Check sheet for the drawn part. Datum: minimum x, y, z corner. Units: mm. A direction names the side the tool comes from. Give positions to 0.01 mm unless a question says otherwise; leave off trailing zeros. Write each loop counter-clockwise with the first axis right and the second up, starting at its lowest first coordinate (ties: lowest second). Pieces come first, ordered by that corner, then holes. Notation, with made-up numbers: M 84,55.5 L 108,55.5 A28 ccw 108,90.5 Z; hole C -13,-27 d4. An arc over 180 degrees is marked long. Write item = value, one per line.
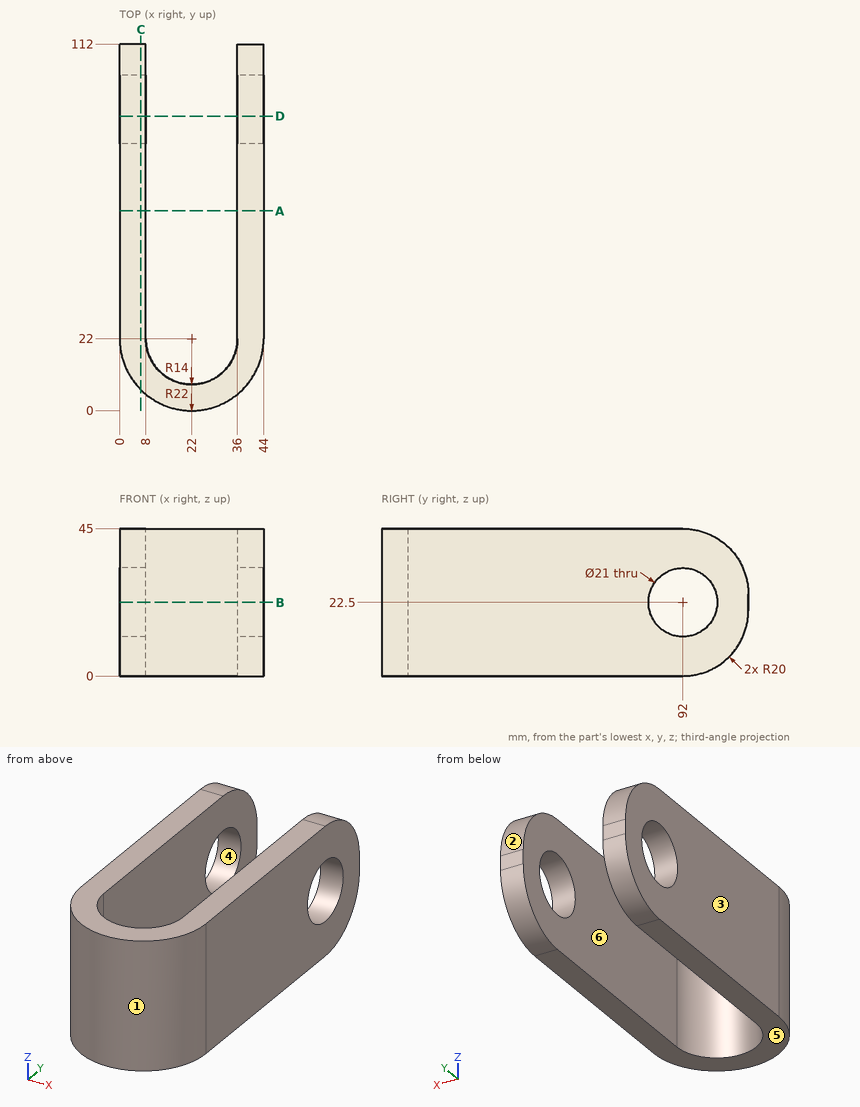
1) Draft check along Y on the marked faces 1, 2, 3 and 4. Enter one of: +Y half, -Y half, draft (parallel to the pull), parting line (faces both ways), or undercut.
From the geometry:
face_1 = -Y half
face_2 = +Y half
face_3 = draft
face_4 = undercut
2) Cross-section at D-D on y = 90. Record the boundary of the cut face in (x, z), plus the area to 3 significant figures.
From the geometry:
outline = M 0,0 L 8,0 L 8,12.19 L 0,12.19 Z; M 0,32.81 L 8,32.81 L 8,45 L 0,45 Z; M 36,0 L 44,0 L 44,12.19 L 36,12.19 Z; M 36,32.81 L 44,32.81 L 44,45 L 36,45 Z
area = 390 mm^2
3) Cross-section at A-A on y = 61. Record the boundary of the cut face in (x, z).
From the geometry:
outline = M 0,0 L 8,0 L 8,45 L 0,45 Z; M 36,0 L 44,0 L 44,45 L 36,45 Z
4) Depth check by flat-ended pin: P1, Ø1.5, axis at x = 31, z = 34.5, coming from the -Y side; P2, Ø6, axis at x = 7.5, z = 10.5, coming from the +Y side; P3, Ø5, axis at x = 38.5, z = 7.5, coming from the -Y side. Enter the tip coordinate at first touch or a pass-through.
From the geometry:
P1 = 1.61
P2 = 110.91
P3 = 5.03
5) Cross-section at C-C on x = 6.5. Record the boundary of the cut face in (y, z).
From the geometry:
outline = M 6.39,0 L 92,0 A20 ccw 112,20 L 112,25 A20 ccw 92,45 L 6.39,45 Z; hole C 92,22.5 d21
6) Tool access check on the marked faces 5 and 6. Record the directions out of +Z, -Z, +X, -X, +Y, -Y that give a thin tool (end or side, any length) a straight path to the whole face; none if there is none.
From the geometry:
face_5 = -Z, +X, -X, +Y, -Y
face_6 = +Z, -Z, +Y
7) Cross-section at B-B on z = 22.5. Record the boundary of the cut face in (x, y), plus the area to 3 significant figures.
From the geometry:
outline = M 0,22 A22 ccw 44,22 L 44,81.5 L 36,81.5 L 36,22 A14 cw 8,22 L 8,81.5 L 0,81.5 Z; M 0,102.5 L 8,102.5 L 8,112 L 0,112 Z; M 36,102.5 L 44,102.5 L 44,112 L 36,112 Z
area = 1,560 mm^2
8) Material ranges on probe 1 along X at (y, z) = (39, 36.5); probe 2 along Z at (x, y) = (3.25, 92); probe 3 along Y at (x, z) = (42, 31), recorded low to high. Write a range as from..to.
From the geometry:
probe_1 = 0..8, 36..44
probe_2 = 0..12, 33..45
probe_3 = 12.83..85.84, 98.16..111.08
